```python
from build123d import *

# Parameters (mm, degrees)
F3_DEPTH = 2.001


with BuildPart() as f1:
    # F0 (on Front) → F1 (revolve)
    with BuildSketch(Plane.XZ):
        with BuildLine():
            Line((-41.9872180451, 0), (-31.5, 0))
            Line((-31.5, 0), (-31.5, 2))
            Line((-31.5, 2), (-35.6538847118, 2))
            ThreePointArc((-35.6538847118, 2), (-39.0084513316, 3.2923211044), (-40.6289470559, 6.5012468828))
            Line((-40.6289470559, 6.5012468828), (-49.1, 91))
            Line((-49.1, 91), (-49.1, 94))
            Line((-49.1, 94), (-51.1, 94))
            Line((-51.1, 94), (-51.1, 91.4))
            ThreePointArc((-51.1, 91.4), (-51.0875233888, 90.9006238306), (-51.0501246883, 90.4024937656))
            Line((-51.0501246883, 90.4024937656), (-41.9872180451, 0))
        make_face()
    revolve(axis=Axis((0, 0, -11.3997804001), (0, 0, -1)))

    # F2 (on face) → F3 (cut, through all)
    with BuildSketch(Plane.XY.offset(2)):
        with BuildLine():
            ThreePointArc((31.5, 0), (31.4841069455, -1.0005047961), (31.4364438192, -2))
            ThreePointArc((31.4364438192, -2), (33.4364438192, 0), (31.4364438192, 2))
            ThreePointArc((31.4364438192, 2), (31.4841069455, 1.0005047961), (31.5, 0))
        make_face()
    extrude(amount=-F3_DEPTH, mode=Mode.SUBTRACT)


solid = f1.part
```
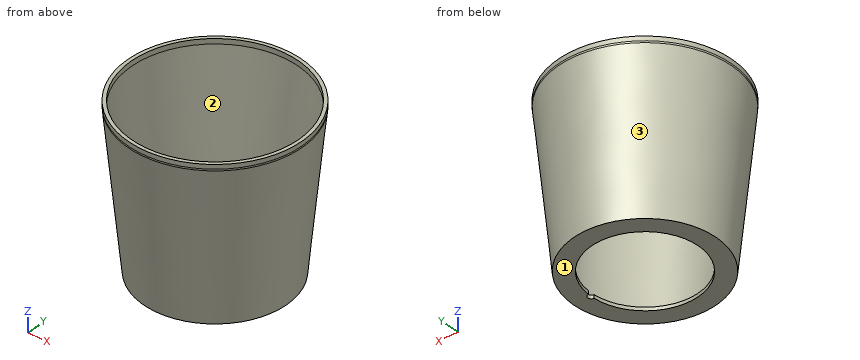
Source: CAD feature listing. Evaluate the final solid. Frame: model axes, mm. Face numbers are marked on the shaded views. Round coordinates to 2 decimals unless told otherwise and drop trailing zeros. Loops run counter-clockwise (first coordinate to the right, second up) from the corner with the lowest first, then second, coordinate; pieces in that order, holes last.
1. Ray query, L1, parallel to Y at x = 0, z = 92; L2, parallel to X at y = 2, z = 11; L3, parallel to X at y = -30, z = 49.5. Return the intervals inside material, ascending.
2. Section query C-C on z = 23.5. Output: boundary loops of the cut face in (x, y), and give its area (3 significant figures).
3. Section query A-A on x = 0. Output: boundary loops of the cut face in (y, z).
4. Mould query, pull axis Y, two halves, no side actions, for the marked faces 1, 2 and 3. Classes: released by +Y, released by -Y, zero draft, split by the parting line, or undercut.
5. Section query B-B on z = 78. Output: boundary loops of the cut face in (x, y), and give its area (3 significant figures).
6. Contact query for flat-ended pins moving along their axis: pin 1 (12 mm diameter, centred on x = -20.5, y = 19.5, fed in from +Z); pin 2 (1.5 mm diameter, centred on y = 24, z = 53, fed in from -X); pin 3 (1 mm diameter, centred on x = 31.5, z = 79, fed in from +Y). Output: stop coordinate, or through.
Answers below:
1. L1: y = -51.1 to -49.1, 49.1 to 51.1
1. L2: x = -43.04 to -41.03, 41.03 to 43.04
1. L3: x = -36.11 to -33.46, 33.46 to 36.11
2. outline: circle Ø88.69 at (0, 0); hole circle Ø84.67 at (0, 0)
2. area: 547 mm2
3. outline: (-51.1, 91.4) arc R10 ccw to (-51.05, 90.4) - (-41.99, 0) - (-31.5, 0) - (-31.5, 2) - (-35.65, 2) arc R5 cw to (-40.63, 6.5) - (-49.1, 91) - (-49.1, 94) - (-51.1, 94) - close; (31.5, 0) - (41.99, 0) - (51.05, 90.4) arc R10 ccw to (51.1, 91.4) - (51.1, 94) - (49.1, 94) - (49.1, 91) - (40.63, 6.5) arc R5 cw to (35.65, 2) - (31.5, 2) - close
4. face 1: zero draft
4. face 2: undercut
4. face 3: split by the parting line
5. outline: circle Ø99.61 at (0, 0); hole circle Ø95.59 at (0, 0)
5. area: 616 mm2
6. pin 1: stops at z = 2
6. pin 2: stops at x = -41.2
6. pin 3: stops at y = 39.12
